Study the drawing (mm; zero at the part's minimum x, y, z) and answer. A direction names the side the tool comes from. Give positions to 0.01 mm unless a question says otherwise; leave off trailing zeros. Write each loop counter-clockwise with the first axis right and the second up, starting at its lowest first coordinate (ties: lowest second). Pieces come first, ordered by that corner, then holes. Notation, with made-up numbers: (65.25, -10.75) -> (90.25, -10.75) arc R21 ccw to (90.25, 18.25) -> close; hole circle Ø1 at (-22.5, -40). An arc over 180 degrees is marked (long way). Put each result on its own line as item: value. Start each with the question number.
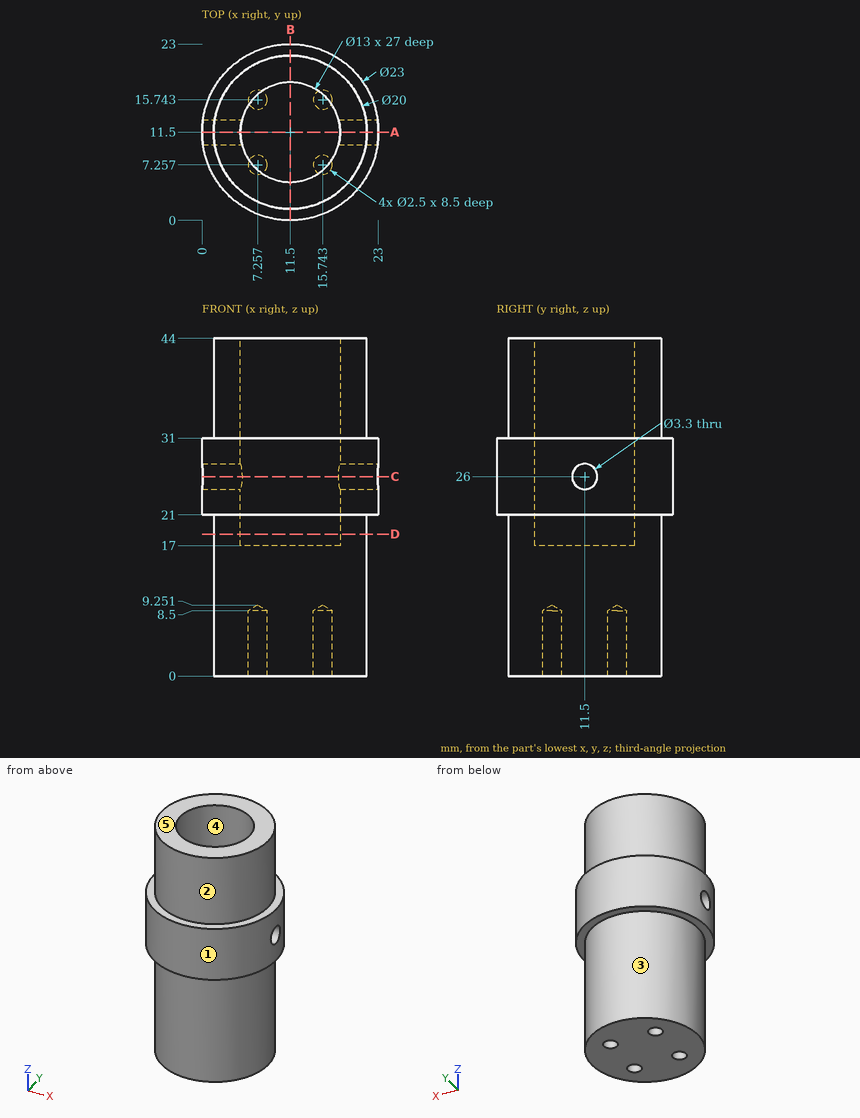
1) Straight lines are drawn through the part: line 1 (Y direction, x = 11.5, z = 39.5); line 2 (Z direction, x = 17, y = 14.75); line 3 (Y direction, x = 2.85, z = 26). For each, find the intervals that lie inside material, in ascending order. Write a range as [from, to].
2) A cutting plane is placed at D-D on z = 18.5. Give the vertices of the cut face in (x, y).
3) For the marked faces 1 and 2, determine the directions among +Z, -Z, +X, -X, +Y, -Y from which every point of the face is accessible in a straight line to the end or side of a thin tool.
4) For a pull along X with two mould halves and no side action, classify the marked faces 3, 4 and 5 as pulls with the +X half, pulls with the -X half, needs draft (parallel to the pull), parting line crosses it, or undercut.
5) Each of these flat-tipped pins is pushed along its axis until it touches: pin 1 Ø8 at (x, z) = (3.5, 5.5) entering from -Y (1 decimal); pin 2 Ø2 at (x, y) = (15.74, 7.26) entering from -Z; pin 3 Ø1 at (x, z) = (13, 23.5) entering from -Y. Where does it stop, or does it pass through?
6) A cutting plane is placed at B-B on x = 11.5. Give the vertices of the cut face in (y, z), and give its area (3 significant figures).
7) A cutting plane is placed at C-C on z = 26. Give the vertices of the cut face in (x, y).
8) A cutting plane is placed at A-A on y = 11.5. Give the vertices of the cut face in (x, z).
Results found:
1. line 1: y = [1.5, 5], [18, 21.5]
1. line 2: z = [0, 17]
1. line 3: y = [3.92, 9.85], [13.15, 19.08]
2. outline: circle Ø20 at (11.5, 11.5); hole circle Ø13 at (11.5, 11.5)
3. face 1: +Z, -Z
3. face 2: +Z
4. face 3: parting line crosses it
4. face 4: undercut
4. face 5: needs draft
5. pin 1: stops at y = 2.3
5. pin 2: stops at z = 8.65
5. pin 3: stops at y = 0.04
6. outline: (0, 21) -> (1.5, 21) -> (1.5, 0) -> (21.5, 0) -> (21.5, 21) -> (23, 21) -> (23, 31) -> (21.5, 31) -> (21.5, 44) -> (18, 44) -> (18, 17) -> (5, 17) -> (5, 44) -> (1.5, 44) -> (1.5, 31) -> (0, 31) -> close
6. area: 559 mm²
7. outline: (0.12, 9.85) arc R11.5 ccw to (22.88, 9.85) -> (17.79, 9.85) arc R6.5 cw to (5.21, 9.85) -> close; (0.12, 13.15) -> (5.21, 13.15) arc R6.5 cw to (17.79, 13.15) -> (22.88, 13.15) arc R11.5 ccw to start
8. outline: (0, 21) -> (1.5, 21) -> (1.5, 0) -> (21.5, 0) -> (21.5, 21) -> (23, 21) -> (23, 24.35) -> (18, 24.35) -> (18, 17) -> (5, 17) -> (5, 24.35) -> (0, 24.35) -> close; (0, 27.65) -> (5, 27.65) -> (5, 44) -> (1.5, 44) -> (1.5, 31) -> (0, 31) -> close; (18, 27.65) -> (23, 27.65) -> (23, 31) -> (21.5, 31) -> (21.5, 44) -> (18, 44) -> close
